Part model, mm, in its own coordinate system. Face numbers are marked on the shaded views. A direction names the side the tool comes from. Give positions to 0.01 mm unless a question says otherwise; leave off trailing zeros. Order: outer loops, then holes, each group sorted by start corner. A loop starts at its lowest first (then second) coordinate and runs counter-clockwise, first axis right, second up. Notation, with made-up numbers: M 20.25,61 L 58.25,61 A14 cw 58.25,72 Z; hole C 27.25,8.5 d6. An arc over 180 degrees is marked long. Answer as a JSON object with one key per item and string values.
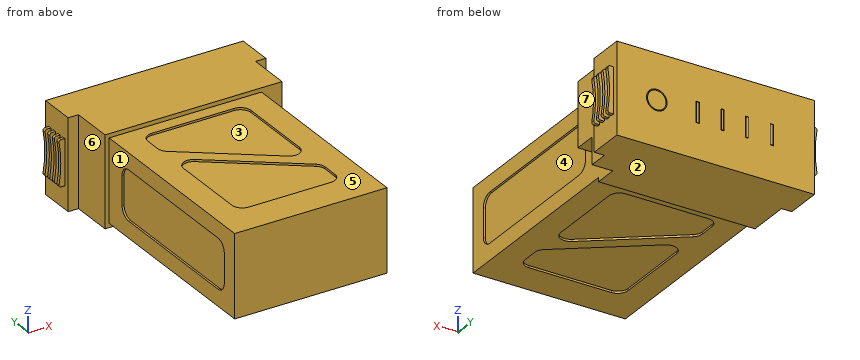
from build123d import *

# Parameters (mm, degrees)
SKETCH_1_W             = 74
SKETCH_1_H             = 40
EXTRUDE_1_DEPTH        = 97
SKETCH_2_W             = 96
SKETCH_2_H             = 44
EXTRUDE_2_DEPTH        = 38
SKETCH_3_W             = 10
SKETCH_3_H             = 13
CUT_EXTRUDE_1_DEPTH    = 11
SKETCH_4_W             = 5
SKETCH_4_H             = 44
CUT_EXTRUDE_2_DEPTH    = 11
SKETCH_5_R             = 5
SKETCH_5_W             = 1.5
SKETCH_5_H             = 10
CUT_EXTRUDE_3_DEPTH    = 2
SKETCH_6_R             = 4.5
SKETCH_6_W             = 1.1
SKETCH_6_H             = 9.6
EXTRUDE_3_DEPTH        = 2
EXTRUDE_4_DEPTH        = 1.6
PATTERN_LINEAR_1_COUNT = 4
PATTERN_LINEAR_1_PITCH = 3.6
MIRROR_2_COPY_1_DEPTH  = 1.6
MIRROR_2_COPY_2_DEPTH  = 1.6
MIRROR_2_COPY_3_DEPTH  = 1.6
CUT_EXTRUDE_4_DEPTH    = 1
CUT_EXTRUDE_5_DEPTH    = 1
SKETCH_10_W            = 5
SKETCH_10_H            = 20.5
SKETCH_10_H_2          = 9.5
CUT_EXTRUDE_6_DEPTH    = 153.199942279


with BuildPart() as part:
    # 草图1 → 凸台-拉伸1 (new body)
    with BuildSketch(Plane(origin=(0, 0, 0), x_dir=(1, 0, 0), z_dir=(0, 1, 0))):
        Rectangle(SKETCH_1_W, SKETCH_1_H)
    extrude(amount=EXTRUDE_1_DEPTH)

    # 草图2 → 凸台-拉伸2 (add)
    with BuildSketch(Plane(origin=(0, 97, 0), x_dir=(1, 0, 0), z_dir=(0, 1, 0))):
        with Locations((4, 0)):
            Rectangle(SKETCH_2_W, SKETCH_2_H)
    extrude(amount=EXTRUDE_2_DEPTH)

    # 草图3 → 切除-拉伸1 (cut)
    with BuildSketch(Plane.XZ.offset(-97)):
        with Locations((42, -15.5)):
            Rectangle(SKETCH_3_W, SKETCH_3_H)
    extrude(amount=-CUT_EXTRUDE_1_DEPTH, mode=Mode.SUBTRACT)

    # 草图4 → 切除-拉伸2 (cut)
    with BuildSketch(Plane.XZ.offset(-97)):
        with Locations((49.5, 0)):
            Rectangle(SKETCH_4_W, SKETCH_4_H)
    extrude(amount=-CUT_EXTRUDE_2_DEPTH, mode=Mode.SUBTRACT)

    # 草图5 → 切除-拉伸3 (cut)
    with BuildSketch(Plane(origin=(0, 135, 0), x_dir=(1, 0, 0), z_dir=(0, 1, 0))):
        with Locations(Location((32.584956569, 0, 0), (0, 0, 270))):
            Circle(SKETCH_5_R)
        with Locations((12.683099686, 0)):
            Rectangle(SKETCH_5_W, SKETCH_5_H)
        with Locations((0.683099686, 0)):
            Rectangle(SKETCH_5_W, SKETCH_5_H)
        with Locations((-11.316900314, 0)):
            Rectangle(SKETCH_5_W, SKETCH_5_H)
        with Locations((-23.316900314, 0)):
            Rectangle(SKETCH_5_W, SKETCH_5_H)
    extrude(amount=-CUT_EXTRUDE_3_DEPTH, mode=Mode.SUBTRACT)

    # 草图6 → 凸台-拉伸3 (add)
    with BuildSketch(Plane(origin=(0, 133, 0), x_dir=(1, 0, 0), z_dir=(0, 1, 0))):
        with Locations(Location((32.584956569, 0, 0), (0, 0, 270))):
            Circle(SKETCH_6_R)
        with Locations((-23.316900314, 0)):
            Rectangle(SKETCH_6_W, SKETCH_6_H)
        with Locations((-11.316900314, 0)):
            Rectangle(SKETCH_6_W, SKETCH_6_H)
        with Locations((0.683099686, 0)):
            Rectangle(SKETCH_6_W, SKETCH_6_H)
        with Locations((12.683099686, 0)):
            Rectangle(SKETCH_6_W, SKETCH_6_H)
    extrude(amount=EXTRUDE_3_DEPTH)

    # 草图7 → 凸台-拉伸4 (add)
    with BuildSketch(Plane(origin=(0, 132.5, 0), x_dir=(1, 0, 0), z_dir=(0, 1, 0))):
        with BuildLine():
            Line((-44, -11.057288531), (-45.807138492, -11.057288531))
            ThreePointArc((-45.807138492, -11.057288531), (-46.570313957, -10.703479841), (-46.793453199, -9.892414949))
            ThreePointArc((-46.793453199, -9.892414949), (-45.972335636, 0), (-46.793453199, 9.892414949))
            ThreePointArc((-46.793453199, 9.892414949), (-46.570313957, 10.703479841), (-45.807138492, 11.057288531))
            Line((-45.807138492, 11.057288531), (-44, 11.057288531))
            Line((-44, 11.057288531), (-44, -11.057288531))
        make_face()
    extrude_4 = extrude(amount=-EXTRUDE_4_DEPTH)

    # 阵列(线性)1: 凸台-拉伸4 ×4
    with Locations(*[(0, -i * PATTERN_LINEAR_1_PITCH, 0) for i in range(1, PATTERN_LINEAR_1_COUNT)]):
        add(extrude_4)

    # 镜向2: 凸台-拉伸4 across plane
    add(extrude_4.mirror(Plane.ZY.offset(-4)))

    # 镜向2 copy 1 sketch → 镜向2 copy 1 (add)
    with BuildSketch(Plane(origin=(8, 128.9, 0), x_dir=(-1, 0, 0), z_dir=(0, 1, 0))):
        with BuildLine():
            Line((-44, 11.057288531), (-45.807138492, 11.057288531))
            ThreePointArc((-45.807138492, 11.057288531), (-46.570313957, 10.703479841), (-46.793453199, 9.892414949))
            ThreePointArc((-46.793453199, 9.892414949), (-45.972335636, 0), (-46.793453199, -9.892414949))
            ThreePointArc((-46.793453199, -9.892414949), (-46.570313957, -10.703479841), (-45.807138492, -11.057288531))
            Line((-45.807138492, -11.057288531), (-44, -11.057288531))
            Line((-44, -11.057288531), (-44, 11.057288531))
        make_face()
    extrude(amount=-MIRROR_2_COPY_1_DEPTH)

    # 镜向2 copy 2 sketch → 镜向2 copy 2 (add)
    with BuildSketch(Plane(origin=(8, 125.3, 0), x_dir=(-1, 0, 0), z_dir=(0, 1, 0))):
        with BuildLine():
            Line((-44, 11.057288531), (-45.807138492, 11.057288531))
            ThreePointArc((-45.807138492, 11.057288531), (-46.570313957, 10.703479841), (-46.793453199, 9.892414949))
            ThreePointArc((-46.793453199, 9.892414949), (-45.972335636, 0), (-46.793453199, -9.892414949))
            ThreePointArc((-46.793453199, -9.892414949), (-46.570313957, -10.703479841), (-45.807138492, -11.057288531))
            Line((-45.807138492, -11.057288531), (-44, -11.057288531))
            Line((-44, -11.057288531), (-44, 11.057288531))
        make_face()
    extrude(amount=-MIRROR_2_COPY_2_DEPTH)

    # 镜向2 copy 3 sketch → 镜向2 copy 3 (add)
    with BuildSketch(Plane(origin=(8, 121.7, 0), x_dir=(-1, 0, 0), z_dir=(0, 1, 0))):
        with BuildLine():
            Line((-44, 11.057288531), (-45.807138492, 11.057288531))
            ThreePointArc((-45.807138492, 11.057288531), (-46.570313957, 10.703479841), (-46.793453199, 9.892414949))
            ThreePointArc((-46.793453199, 9.892414949), (-45.972335636, 0), (-46.793453199, -9.892414949))
            ThreePointArc((-46.793453199, -9.892414949), (-46.570313957, -10.703479841), (-45.807138492, -11.057288531))
            Line((-45.807138492, -11.057288531), (-44, -11.057288531))
            Line((-44, -11.057288531), (-44, 11.057288531))
        make_face()
    extrude(amount=-MIRROR_2_COPY_3_DEPTH)

    # 草图8 → 切除-拉伸4 (cut)
    with BuildSketch(Plane.ZY.offset(37)):
        with BuildLine():
            Line((-7, 87), (7, 87))
            ThreePointArc((7, 87), (10.535533906, 85.535533906), (12, 82))
            Line((12, 82), (12, 13))
            ThreePointArc((12, 13), (10.535533906, 9.464466094), (7, 8))
            Line((7, 8), (-7, 8))
            ThreePointArc((-7, 8), (-10.535533906, 9.464466094), (-12, 13))
            Line((-12, 13), (-12, 82))
            ThreePointArc((-12, 82), (-10.535533906, 85.535533906), (-7, 87))
        make_face()
    cut_extrude_4 = extrude(amount=-CUT_EXTRUDE_4_DEPTH, mode=Mode.SUBTRACT)

    # 镜向3: 切除-拉伸4 across plane
    add(cut_extrude_4.mirror(Plane(origin=(0, 0, 0), x_dir=(0, 0, 1), z_dir=(1, 0, 0))), mode=Mode.SUBTRACT)

    # 草图9 → 切除-拉伸5 (cut)
    with BuildSketch(Plane(origin=(0, 0, -20), x_dir=(-1, 0, 0), z_dir=(0, 0, -1))):
        with BuildLine():
            Line((-20, 91.06721858), (20, 91.06721858))
            ThreePointArc((20, 91.06721858), (23.535533906, 89.602752486), (25, 86.06721858))
            Line((25, 86.06721858), (25, 78.57061248))
            ThreePointArc((25, 78.57061248), (24.470921387, 76.332117014), (22.995655219, 74.567357579))
            Line((22.995655219, 74.567357579), (-17.004344781, 44.635161975))
            ThreePointArc((-17.004344781, 44.635161975), (-22.238495466, 44.167495489), (-25, 48.638416876))
            Line((-25, 48.638416876), (-25, 86.06721858))
            ThreePointArc((-25, 86.06721858), (-23.535533906, 89.602752486), (-20, 91.06721858))
        make_face()
        with BuildLine():
            Line((-22.995655219, 32.657933054), (17.004344781, 62.590128658))
            ThreePointArc((17.004344781, 62.590128658), (22.238495466, 63.057795143), (25, 58.586873756))
            Line((25, 58.586873756), (25, 21.158072053))
            ThreePointArc((25, 21.158072053), (23.535533906, 17.622538147), (20, 16.158072053))
            Line((20, 16.158072053), (-20, 16.158072053))
            ThreePointArc((-20, 16.158072053), (-23.535533906, 17.622538147), (-25, 21.158072053))
            Line((-25, 21.158072053), (-25, 28.654678152))
            ThreePointArc((-25, 28.654678152), (-24.470921387, 30.893173618), (-22.995655219, 32.657933054))
        make_face()
    cut_extrude_5 = extrude(amount=-CUT_EXTRUDE_5_DEPTH, mode=Mode.SUBTRACT)

    # 镜向4: 切除-拉伸5 across plane
    add(cut_extrude_5.mirror(Plane.XY), mode=Mode.SUBTRACT)

    # 草图10 → 切除-拉伸6 (cut, through all)
    with BuildSketch(Plane(origin=(0, 0, -22), x_dir=(-1, 0, 0), z_dir=(0, 0, -1))):
        with Locations((41.5, 107.25)):
            Rectangle(SKETCH_10_W, SKETCH_10_H)
        with Locations((-49.5, 112.75)):
            Rectangle(SKETCH_10_W, SKETCH_10_H_2)
    extrude(amount=-CUT_EXTRUDE_6_DEPTH, mode=Mode.SUBTRACT)


solid = part.part
1. Cut at D-D on y = 111.5. Give the cut face in (x, z).
Worked answers:
{"outline": "M -39,-22 L 47,-22 L 47,22 L -39,22 Z"}
2. Cut at C-C on y = 42. Give the cut face in (x, z).
Worked answers:
{"outline": "M -37,-20 L -25,-20 L -25,-19 L 10.51,-19 L 10.51,-20 L 37,-20 L 37,-12 L 36,-12 L 36,12 L 37,12 L 37,20 L 10.51,20 L 10.51,19 L -25,19 L -25,20 L -37,20 L -37,12 L -36,12 L -36,-12 L -37,-12 Z"}
3. Cut at B-B on x = -2. Give the cut face in (y, z).
Worked answers:
{"outline": "M 0,-20 L 16.16,-20 L 16.16,-19 L 51.36,-19 L 51.36,-20 L 58.86,-20 L 58.86,-19 L 91.07,-19 L 91.07,-20 L 97,-20 L 97,-22 L 135,-22 L 135,22 L 97,22 L 97,20 L 91.07,20 L 91.07,19 L 58.86,19 L 58.86,20 L 51.36,20 L 51.36,19 L 16.16,19 L 16.16,20 L 0,20 Z"}
4. Which spindle directions (+Z, -Z, +X, -X, +Y, -Y) get a long thin tool onto all of the face, cutting with end or side? Do the marked faces 4, 5, 6 and 7. Say none if no direction does.
Worked answers:
{"face 4": "+X", "face 5": "+Z, +X, -X, -Y", "face 6": "+Z, -Z, -X, -Y", "face 7": "+Z, -Z, +X, -Y"}
5. Pin check, flat tips, straight feed: P1, Ø1.5, axis at x = 22, y = 90, coming from the +Z side; P2, Ø2, axis at y = 134.5, z = 0, coming from the +X side; P3, Ø2, axis at x = 53.5, z = 5, coming from the -Y side. Stop position of each tip, or through.
Worked answers:
{"P1": "stops at z = 20", "P2": "stops at x = 52", "P3": "stops at y = 120.1"}
6. Probe line 1 along Z through (x, y) = (-3.5, 74); line 2 along X through (y, z) = (118.5, 3.5); line 3 along Z through (x, y) = (-1, 57). List the from-to ranges inside material, lowest first.
Worked answers:
{"line 1": "z = -19 to 19", "line 2": "x = -44 to 52", "line 3": "z = -20 to 20"}
7. Cut at A-A on y = 24.5. Give the cut face in (x, z), plus the area to 3 significant figures.
Worked answers:
{"outline": "M -37,-20 L -25,-20 L -25,-19 L 25,-19 L 25,-20 L 37,-20 L 37,-12 L 36,-12 L 36,12 L 37,12 L 37,20 L 25,20 L 25,19 L -25,19 L -25,20 L -37,20 L -37,12 L -36,12 L -36,-12 L -37,-12 Z", "area": "2,810 mm^2"}
8. Two-plate mould, pull along X, no slides. Class the marked faces 1, 2 and 3: +X half, -X half, draft (parallel to the pull), parting line (faces both ways), or undercut.
Worked answers:
{"face 1": "-X half", "face 2": "draft", "face 3": "undercut"}
